```python
from build123d import *

# Parameters (mm, degrees)
SKETCH_1_R      = 2.475
EXTRUDE_1_DEPTH = 16
SKETCH_2_R      = 3.75
EXTRUDE_2_DEPTH = 4
CHAMFER_1_SIZE  = 0.5
EXTRUDE_3_DEPTH = 2
CHAMFER_2_SIZE  = 0.1
FILLET_1_R      = 1


# Read off the part's stored shape, not the designer's step: the extrude step
with BuildPart() as part:
    # 스케치1 → 보스-돌출1 (new body)
    with BuildSketch(Plane.XY):
        Circle(SKETCH_1_R)
    extrude(amount=EXTRUDE_1_DEPTH)

    # 스케치2 → 보스-돌출2 (add)
    with BuildSketch(Plane.XY.offset(16)):
        Circle(SKETCH_2_R)
    extrude(amount=EXTRUDE_2_DEPTH)

    # 모따기1
    chamfer_1_edges = [part.edges().sort_by_distance(p)[0] for p in [
        (-3.75, 0, 16),
        (-3.75, 0, 20),
    ]]
    chamfer(chamfer_1_edges, length=CHAMFER_1_SIZE)

    # 보스-돌출3 outline → 보스-돌출3 (add)
    with BuildSketch(Plane.XY.offset(20)):
        with BuildLine():
            ThreePointArc((2.883140649, -1.5), (2.974111162, -1.310405585), (3.05263006, -1.115324937))
            Line((3.05263006, -1.115324937), (3.05263006, 1.115324937))
            ThreePointArc((3.05263006, 1.115324937), (2.974111162, 1.310405585), (2.883140649, 1.5))
            Line((2.883140649, 1.5), (-2.883140649, 1.5))
            ThreePointArc((-2.883140649, 1.5), (-2.974111162, 1.310405585), (-3.05263006, 1.115324937))
            Line((-3.05263006, 1.115324937), (-3.05263006, -1.115324937))
            ThreePointArc((-3.05263006, -1.115324937), (-2.974111162, -1.310405585), (-2.883140649, -1.5))
            Line((-2.883140649, -1.5), (2.883140649, -1.5))
        make_face()
    extrude(amount=EXTRUDE_3_DEPTH)

    # 모따기2
    chamfer_2_edges = [part.edges().sort_by_distance(p)[0] for p in [
        (3.05263006, 0, 22),
        (-3.05263006, 0, 22),
        (0, -1.5, 22),
        (0, 1.5, 22),
    ]]
    chamfer(chamfer_2_edges, length=CHAMFER_2_SIZE)

    # 필렛1
    fillet_1_edges = [part.edges().sort_by_distance(p)[0] for p in [
        (-2.475, 0, 0),
    ]]
    fillet(fillet_1_edges, radius=FILLET_1_R)


solid = part.part
```
Source: CAD feature listing. Evaluate the final solid. Frame: model axes, mm. A direction names the side the tool comes from. Round coordinates to 2 decimals unless told otherwise and drop trailing zeros. Order: outer loops, then holes, each group sorted by start corner. A loop starts at its lowest first (then second) coordinate and runs counter-clockwise, first axis right, second up. Notation, with made-up numbers: (89.25, 84.25) -> (119.25, 84.25) arc R7 ccw to (119.25, 94.25) -> close; hole circle Ø5 at (80.25, 85). An arc over 180 degrees is marked (long way). Use CSV: the item, a comma, the result in double quotes.
(1) Access query for faces 1 (the face through (0, 2, 20)), 2 (the face through (-3.053, 0, 21)), 3 (the face through (3.053, 0, 21)), 4 (the face through (0, -2, 20)). Directions: +Z, -Z, +X, -X, +Y, -Y. A direction counts if a zero-diameter tool reaches every point of the face in a straight line with its end or side. Return the directions, or none.
Report:
face 1,"+Z, +X, -X, +Y"
face 2,"+Z, -X, +Y, -Y"
face 3,"+Z, +X, +Y, -Y"
face 4,"+Z, +X, -X, -Y"
(2) Ray query, L1, parallel to Z at x = 2.5, y = 2; L2, parallel to Y at x = 0, z = 2 (3 decimals); L3, parallel to Z at x = -2.75, y = -1. Return the intervals inside material, ascending.
Report:
L1,"16 to 20"
L2,"-2.475 to 2.475"
L3,"16 to 22"
(3) Section B-B on z = 20.5. Return the cut outline in (x, y).
Report:
outline,"(-3.05, -1.12) arc R3.25 ccw to (-2.88, -1.5) -> (2.88, -1.5) arc R3.25 ccw to (3.05, -1.12) -> (3.05, 1.12) arc R3.25 ccw to (2.88, 1.5) -> (-2.88, 1.5) arc R3.25 ccw to (-3.05, 1.12) -> close"
(4) First-contact query: pin 1 Ø3 at (y, z) = (-1.5, 6) entering from -X (3 decimals); pin 2 Ø1.5 at (x, z) = (-0.5, 21) entering from -Y; pin 3 Ø1.5 at (x, y) = (1.5, -2.5) entering from -Z. Flat tips, straight axial feed; report the tip coordinate or a pass-through.
Report:
pin 1,"x = -2.475"
pin 2,"y = -1.5"
pin 3,"z = 0.28"
(5) Section A-A on x = 0. Return the cut outline in (y, z) (3 decimals), and give its area (3 significant figures).
Report:
outline,"(-3.75, 16.5) -> (-3.25, 16) -> (-2.475, 16) -> (-2.475, 1) arc R1 ccw to (-1.475, 0) -> (1.475, 0) arc R1 ccw to (2.475, 1) -> (2.475, 16) -> (3.25, 16) -> (3.75, 16.5) -> (3.75, 19.5) -> (3.25, 20) -> (1.5, 20) -> (1.5, 21.9) -> (1.4, 22) -> (-1.4, 22) -> (-1.5, 21.9) -> (-1.5, 20) -> (-3.25, 20) -> (-3.75, 19.5) -> close"
area,"114 mm^2"
(6) Section C-C on z = 10.75. Return the cut outline in (x, y) (3 decimals), and give its area (3 significant figures).
Report:
outline,"circle Ø4.95 at (0, 0)"
area,"19.2 mm^2"
